CAD build for the part. Positions are in the model's coordinates, mm. A direction names the side the tool comes from. Round coordinates to 2 decimals unless told otherwise and drop trailing zeros. Loops run counter-clockwise (first coordinate to the right, second up) from the corner with the lowest first, then second, coordinate; pieces in that order, holes last.
from build123d import *

# Parameters (mm, degrees)
SKETCH1_R                      = 3.6
SKETCH1_R_2                    = 2.55
BOSS_EXTRUDE1_DEPTH            = 6
M5X0_8_TAPPED_HOLE1_D          = 4.2
SKETCH2_R                      = 6
SKETCH2_R_2                    = 5.05
CUT_EXTRUDE1_DEPTH             = 2
SKETCH5_W                      = 5.25
SKETCH5_H                      = 6.7
CUT_EXTRUDE2_DEPTH             = 2.18
SKETCH6_W                      = 2.5
SKETCH6_H                      = 6.7
CUT_EXTRUDE3_DEPTH             = 4.82
CBORE_FOR_M5_SHCS1_D           = 5.5
CBORE_FOR_M5_SHCS1_CBORE_D     = 10
CBORE_FOR_M5_SHCS1_CBORE_DEPTH = 3.2


with BuildPart() as part:
    # Sketch1 → Boss-Extrude1 (new body)
    with BuildSketch(Plane(origin=(0, 0, 0), x_dir=(1, 0, 0), z_dir=(0, 1, 0))):
        with BuildLine():
            Line((20.365, -25), (-20.365, -25))
            ThreePointArc((-20.365, -25), (-23.642439931, -23.642439931), (-25, -20.365))
            Line((-25, -20.365), (-25, 20.365))
            ThreePointArc((-25, 20.365), (-23.642439931, 23.642439931), (-20.365, 25))
            Line((-20.365, 25), (20.365, 25))
            ThreePointArc((20.365, 25), (23.642439931, 23.642439931), (25, 20.365))
            Line((25, 20.365), (25, -20.365))
            ThreePointArc((25, -20.365), (23.642439931, -23.642439931), (20.365, -25))
        make_face()
        with Locations((-15, 15.95)):
            Circle(SKETCH1_R, mode=Mode.SUBTRACT)
        with Locations((15, 15.95)):
            Circle(SKETCH1_R, mode=Mode.SUBTRACT)
        with Locations((15, -15.95)):
            Circle(SKETCH1_R_2, mode=Mode.SUBTRACT)
        with Locations((-15, -15.95)):
            Circle(SKETCH1_R_2, mode=Mode.SUBTRACT)
    extrude(amount=BOSS_EXTRUDE1_DEPTH)

    # M5x0.8 Tapped Hole1 (through all)
    with Locations(Plane(origin=(0, 6, 0), x_dir=(1, 0, 0), z_dir=(0, 1, 0))):
        with Locations((0, 10), (-10, 0), (0, 0), (0, -10), (10, 0)):
            Hole(M5X0_8_TAPPED_HOLE1_D / 2)

    # Sketch2 → Cut-Extrude1 (cut)
    with BuildSketch(Plane(origin=(0, 6, 0), x_dir=(1, 0, 0), z_dir=(0, 1, 0))):
        with Locations((-15, 15.95)):
            Circle(SKETCH2_R)
        with Locations((15, 15.95)):
            Circle(SKETCH2_R)
        with Locations((15, -15.95)):
            Circle(SKETCH2_R_2)
        with Locations((-15, -15.95)):
            Circle(SKETCH2_R_2)
    extrude(amount=-CUT_EXTRUDE1_DEPTH, mode=Mode.SUBTRACT)

    # Sketch5 → Cut-Extrude2 (cut)
    with BuildSketch(Plane(origin=(0, 6, 0), x_dir=(1, 0, 0), z_dir=(0, 1, 0))):
        with Locations((-22.375, 0)):
            Rectangle(SKETCH5_W, SKETCH5_H)
        with Locations((22.375, 0)):
            Rectangle(SKETCH5_W, SKETCH5_H)
    extrude(amount=-CUT_EXTRUDE2_DEPTH, mode=Mode.SUBTRACT)

    # Sketch6 → Cut-Extrude3 (cut, through all)
    with BuildSketch(Plane(origin=(0, 3.82, 0), x_dir=(1, 0, 0), z_dir=(0, 1, 0))):
        with Locations((-21, 0)):
            Rectangle(SKETCH6_W, SKETCH6_H)
        with Locations((21, 0)):
            Rectangle(SKETCH6_W, SKETCH6_H)
    extrude(amount=-CUT_EXTRUDE3_DEPTH, mode=Mode.SUBTRACT)

    # CBORE for M5 SHCS1 (through all)
    with Locations(Plane(origin=(0, 0, 0), x_dir=(-1, 0, 0), z_dir=(0, -1, 0))):
        with Locations((0, 10), (0, -10)):
            CounterBoreHole(CBORE_FOR_M5_SHCS1_D / 2, CBORE_FOR_M5_SHCS1_CBORE_D / 2, CBORE_FOR_M5_SHCS1_CBORE_DEPTH)


solid = part.part
Item 1: 3-axis set-ups, long thin cutter, end or side, ignore diameter. For faces 4 (the flat face through (-2.2, 3.2, 12.2)), 5 (the cylindrical face through (-11.774, 5.014, -21.009)), 6 (the flat face through (19.75, 3, 0)), 7 (the flat face through (24, 3.82, 0)): which of +Z, -Z, +X, -X, +Y, -Y reach the whole face in a straight line?
Verdict:
face 4: -Y
face 5: +Y
face 6: +Y, -Y
face 7: +X, +Y
Item 2: Cut at B-B (x = 0). List the corners of the cut face in (y, z).
Verdict:
outline: (0, -25) - (6, -25) - (6, -12.75) - (3.2, -12.75) - (3.2, -15) - (0, -15) - close; (0, -5) - (3.2, -5) - (3.2, -7.25) - (6, -7.25) - (6, -2.1) - (0, -2.1) - close; (0, 2.1) - (6, 2.1) - (6, 7.25) - (3.2, 7.25) - (3.2, 5) - (0, 5) - close; (0, 15) - (3.2, 15) - (3.2, 12.75) - (6, 12.75) - (6, 25) - (0, 25) - close
Item 3: Cut at A-A (z = 15.95). List the corners of the cut face in (x, y).
Verdict:
outline: (-25, 0) - (-17.55, 0) - (-17.55, 4) - (-20.05, 4) - (-20.05, 6) - (-25, 6) - close; (-12.45, 0) - (12.45, 0) - (12.45, 4) - (9.95, 4) - (9.95, 6) - (-9.95, 6) - (-9.95, 4) - (-12.45, 4) - close; (17.55, 0) - (25, 0) - (25, 6) - (20.05, 6) - (20.05, 4) - (17.55, 4) - close
Item 4: Mould opens along Z. For faces 1 (the cylindrical face through (23.606, 2.958, -23.678)), 2 (the cylindrical face through (-17.024, 1.972, 17.502)), 3 (the flat face through (-25, 3, 0)) say: released by +Z, released by -Z, zero draft, split by the parting line, or undercut.
Verdict:
face 1: released by -Z
face 2: undercut
face 3: zero draft
Item 5: Flat gauge pins, fed straight in: P1, Ø9.5, axis at x = -15, z = -15.95, coming from the +Y side; P2, Ø9, axis at x = 0, z = 10, coming from the +Y side; P3, Ø0.8, axis at x = -23.5, z = 1.5, coming from the +Y side; P4, Ø7, axis at x = 0, z = -10, coming from the -Y side. Where does each tip first touch, or does it go through?
Verdict:
P1: stops at y = 4
P2: stops at y = 6
P3: stops at y = 3.82
P4: stops at y = 3.2
Item 6: Cut at D-D (x = 15). List the corners of the cut face in (y, z), plus the area to 3 significant figures.
Verdict:
outline: (0, -25) - (6, -25) - (6, -21.95) - (4, -21.95) - (4, -19.55) - (0, -19.55) - close; (0, -12.35) - (4, -12.35) - (4, -9.95) - (6, -9.95) - (6, 10.9) - (4, 10.9) - (4, 13.4) - (0, 13.4) - close; (0, 18.5) - (4, 18.5) - (4, 21) - (6, 21) - (6, 25) - (0, 25) - close
area: 207 mm2
Item 7: Cut at C-C (z = 10). List the corners of the cut face in (x, y).
Verdict:
outline: (-25, 0) - (-5, 0) - (-5, 3.2) - (-2.75, 3.2) - (-2.75, 6) - (-25, 6) - close; (2.75, 3.2) - (5, 3.2) - (5, 0) - (25, 0) - (25, 6) - (2.75, 6) - close
Item 8: Wall check: L1, parallel to X at y = 5.2, z = 15.95; L2, parallel to Z at x = 15, y = 5.5; L3, parallel to X at y = 2.8, z = 15.95. Give the ranges that are in metal, low to high.
Verdict:
L1: x = -25 to -20.05, -9.95 to 9.95, 20.05 to 25
L2: z = -25 to -21.95, -9.95 to 10.9, 21 to 25
L3: x = -25 to -17.55, -12.45 to 12.45, 17.55 to 25
